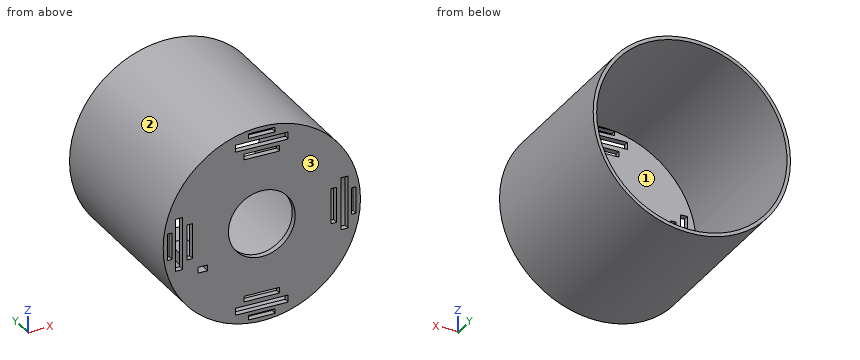
Autodesk Inventor part; units mm, degrees
ref_plane "YZ Plane" through (0, 0, 0) normal (1, 0, 0) x (0, 1, 0)
ref_plane "XZ Plane" through (0, 0, 0) normal (0, 1, 0) x (-1, 0, 0)
ref_plane "XY Plane" through (0, 0, 0) normal (0, 0, 1) x (1, 0, 0)
sketch "Sketch1" plane through (0, 0, 0) normal (0, 1, 0) x (-1, 0, 0)
  circle A0 centre (0, 0) radius 49.1
  dimension "d12" = 98.2
extrude "Extrusion1" add sketch "Sketch1" along normal blind 3
mirror "Mirror1" about plane through (0, 0, 0) normal (0, 0, 1)
sketch "Sketch10" plane through (0, 3, 0) normal (0, 1, 0) x (1, 0, 0)
  circle A0 centre (0, 0) radius 49.1
  circle A1 centre (0, 0) radius 50.9
  dimension "d23" = 101.8
  dimension "d52" = 1.8
extrude "Extrusion4" add sketch "Sketch10" along normal blind 90 and the other way blind 3
sketch "Sketch13" plane through (0, 3, 0) normal (0, 1, 0) x (1, 0, 0)
  line L0 (-35, 13.5) -> (-26, 13.5)
  line L1 (-26, 13.5) -> (-26, 19.5)
  line L2 (-26, 19.5) -> (-35, 19.5)
  line L3 (-35, 19.5) -> (-35, 13.5)
  line L4 (-28, 14.5) -> (-33, 14.5)
  line L5 (-33, 14.5) -> (-33, 17.5)
  line L6 (-33, 17.5) -> (-28, 17.5)
  line L7 (-28, 17.5) -> (-28, 14.5)
  line L8 (0, 0) -> (0, 20.276) construction
  line L9 (-35, 13.5) -> (0, 13.5) construction
  dimension "d31" = 9
  dimension "d32" = 6
  dimension "d33" = 3
  dimension "d35" = 5
  dimension "d36" = 2
  dimension "d54" = 13.5
  dimension "d58" = 26
extrude "Extrusion6" add sketch "Sketch13" along normal blind 20
sketch "Sketch14" plane through (0, 3, 0) normal (0, 1, 0) x (1, 0, 0)
  line L0 (-33, 17.5) -> (-28, 17.5)
  line L1 (-28, 14.5) -> (-33, 14.5)
  line L2 (-33, 17.5) -> (-28, 17.5)
  line L3 (-28, 17.5) -> (-28, 14.5)
  line L4 (-28, 14.5) -> (-33, 14.5)
  line L5 (-33, 14.5) -> (-33, 17.5)
  point P0 (0, 0)
extrude "Extrusion7" cut sketch "Sketch14" against normal blind 5
sketch "Sketch15" plane through (0, 23, 0) normal (0, 1, 0) x (1, 0, 0)
  line L0 (-35, 19.5) -> (-35, 13.5)
  line L1 (-35, 19.5) -> (-26, 19.5)
  line L2 (-26, 19.5) -> (-26, 13.5)
  line L3 (-26, 13.5) -> (-35, 13.5)
  line L4 (-35, 13.5) -> (-35, 19.5)
  point P0 (0, 0)
extrude "Extrusion8" add sketch "Sketch15" along normal blind 2
sketch "Sketch17" plane through (0, 3, 0) normal (0, 1, 0) x (1, 0, 0)
  line L0 (48.6808, -6.9203) -> (46.2945, -6.9203)
  line L1 (46.2945, -6.9203) -> (46.2945, 6.9203)
  line L2 (46.2945, 6.9203) -> (48.6808, 6.9203)
  line L3 (48.6808, 6.9203) -> (48.6808, -6.9203)
  line L4 (48.6808, -6.9203) -> (46.2945, 6.9203) construction
  line L5 (46.2945, -6.9203) -> (48.6808, 6.9203) construction
  line L6 (44.5001, -13.602) -> (40.806, -13.602)
  line L7 (40.806, -13.602) -> (40.806, 13.602)
  line L8 (40.806, 13.602) -> (44.5001, 13.602)
  line L9 (44.5001, 13.602) -> (44.5001, -13.602)
  line L10 (44.5001, -13.602) -> (40.806, 13.602) construction
  line L11 (40.806, -13.602) -> (44.5001, 13.602) construction
  line L12 (38.6361, -9.1592) -> (35.6953, -9.1592)
  line L13 (35.6953, -9.1592) -> (35.6953, 9.1592)
  line L14 (35.6953, 9.1592) -> (38.6361, 9.1592)
  line L15 (38.6361, 9.1592) -> (38.6361, -9.1592)
  line L16 (38.6361, -9.1592) -> (35.6953, 9.1592) construction
  line L17 (35.6953, -9.1592) -> (38.6361, 9.1592) construction
  point P0 (0, 0)
  point P1 (47.4877, 0)
  point P2 (42.6531, 0)
  point P3 (37.1657, 0)
extrude "Extrusion10" cut sketch "Sketch17" against normal blind 5
pattern_circular "Circular Pattern1" count 4 over 360 about axis through (0, -10, 0) along (0, 1, 0) of "Extrusion10"
sketch "Sketch18" plane through (0, 3, 0) normal (0, 1, 0) x (1, 0, 0)
  circle A0 centre (0, 0) radius 17.25
  dimension "d55" = 34.5
extrude "Extrusion11" cut sketch "Sketch18" against normal blind 10
ref_plane "Work Plane1" through (0, 0, 0) normal (0, 0, 1) x (1, 0, 0)
properties part number "Base"
Source: CAD feature listing. Evaluate the final solid. Frame: model axes, mm. Face numbers are marked on the shaded views. Round coordinates to 2 decimals unless told otherwise and drop trailing zeros. Write each loop counter-clockwise with the first axis right and the second up, starting at its lowest first coordinate (ties: lowest second). Pieces come first, ordered by that corner, then holes. Notation, with made-up numbers: M 21,34.5 L 74,34.5 A20 ccw 74,70.5 Z; hole C 67.5,46 d5. An arc over 180 degrees is marked long. One line per item, written item: value. Start each with the question number.
Item 1: Section query B-B (z = -43). Return the cut outline in (x, y), plus the area to 3 significant figures.
Item 2: Mould query, pull axis Z, two halves, no side actions, for the marked faces 1, 2 and 3. Classes: pulls with the +Z half, pulls with the -Z half, needs draft (parallel to the pull), parting line crosses it, or undercut.
Item 3: Section query A-A (y = 6.5). Return the cut outline in (x, z), plus the area to 3 significant figures.
Item 4: Pin query (flat end, axial travel): pin 1 (5 mm diameter, centred on x = 4.5, z = 27, fed in from +Y); pin 2 (1.5 mm diameter, centred on y = 2, z = 1.5, fed in from +X); pin 3 (6 mm diameter, centred on x = -11, y = 60, fed in from -Z). Return the tip coordinate at first contact, or that it passes through.
Item 5: Ray query, L1, parallel to Z at x = 0, y = 29; L2, parallel to Y at x = -31, z = 1.5. Return the intervals inside material, ascending. Write a range as from..to.
Item 6: Section query C-C (x = 0). State how many separate pieces and enclosed holes the cut face has, plus the area to 3 significant figures.
Result set:
1. outline: M -27.24,0 L -13.6,0 L -13.6,3 L -23.7,3 L -23.7,93 L -27.24,93 Z; M 13.6,0 L 27.24,0 L 27.24,93 L 23.7,93 L 23.7,3 L 13.6,3 Z
1. area: 718 mm²
2. face 1: undercut
2. face 2: parting line crosses it
2. face 3: needs draft
3. outline: C 0,0 d101.8; M -35,-19.5 L -26,-19.5 L -26,-13.5 L -35,-13.5 Z; hole C 0,0 d98.2; hole M -33,-17.5 L -28,-17.5 L -28,-14.5 L -33,-14.5 Z
3. area: 604 mm²
4. pin 1: stops at y = 3
4. pin 2: stops at x = 50.89
4. pin 3: stops at z = -50.27
5. L1: z = -50.9..-49.1, 49.1..50.9
5. L2: y = 0..3
6. separate pieces: 8
6. enclosed holes: 0
6. area: 472 mm²
